Geometry: final body of the model. Coordinates: model frame, mm. A direction names the side the tool comes from. Coordinates: 2 decimals unless noted, no trailing zeros. Loops run counter-clockwise (first coordinate to the right, second up) from the corner with the lowest first, then second, coordinate; pieces in that order, holes last. Notation, with made-up numbers: (9.5, -1) - (16.5, -1) arc R21 cw to (16.5, 20) - close; hole circle Ø10 at (-11.5, 36). An arc over 180 degrees is marked (long way). Put each result on its own line as item: value. Start each with the question number.
1) Draft query along Y for faces 1 (the cylindrical face through (-23, -2, -5)), 2 (the flat face through (4, -130, -2)), 3 (the cylindrical face through (-25.479, -79.547, -16.284)). Return one class per face: +Y half, -Y half, draft (parallel to the pull), parting line (faces both ways), or undercut.
2) Section D-D on x = -15.5. Output: boundary loops of the cut face in (y, z), and give its area (3 significant figures).
3) Section C-C on y = -98. Output: boundary loops of the cut face in (x, z), and give its area (3 significant figures).
4) Section B-B on z = -17. Count the separate pieces of the cut face and the enclosed holes in it, and give its area (3 significant figures).
5) Contact query for flat-ended pins moving along their axis: pin 1 Ø19 at (x, y) = (-4.5, 22.5) entering from -Z; pin 2 Ø0.9 at (x, y) = (26, -9) entering from +Z; pin 3 Ø6 at (x, z) = (-18.5, -14) entering from +Y; pin 4 Ø0.9 at (x, y) = (-25.5, 12) entering from +Z. Output: stop coordinate, or through.
6) Section A-A on y = -19.5. Output: boundary loops of the cut face in (x, z).
7) Reachability of faces 4 (the flat face through (27, 2, -24)), 5 (the cylindrical face through (25.5, 115.5, -16.9)), 6 (the cylindrical face through (23, 2, -5)) from +Z, -Z, +X, -X, +Y, -Y: full face, straight path, thin tool, end or side. Return the list, or none.
8) Material intervals for line 1 along Y through (x, z) = (-25.05, -17); line 2 along X through (y, z) = (-66.5, -29.5); line 3 along Z through (x, y) = (-10, 23), sorted ascending. Write a range as from..to.
```python
from build123d import *

# Parameters (mm, degrees)
SKETCH1_W                      = 54
SKETCH1_H                      = 260
BASE_FLANGE1_DEPTH             = 3
EDGE_FLANGE1_STRIP_W           = 22
EDGE_FLANGE1_STRIP_H           = 3
EDGE_FLANGE1_STRIP_CUT_DEPTH   = 260
EDGE_FLANGE1_STRIP_2_W         = 22
EDGE_FLANGE1_STRIP_2_H         = 3
EDGE_FLANGE1_STRIP_CUT_2_DEPTH = 260
EDGE_FLANGE1_DEPTH             = 260
EDGE_FLANGE1_BEND_DEPTH        = 260
CUT_EXTRUDE1_DEPTH             = 145.817126059
SKETCH20_R                     = 5.5
CUT_EXTRUDE2_DEPTH             = 145.817126059


# Sheet-metal steps are written as plain solids
with BuildPart() as part:
    # Sketch1 → Base-Flange1 (new body)
    with BuildSketch(Plane.XY):
        Rectangle(SKETCH1_W, SKETCH1_H)
    extrude(amount=-BASE_FLANGE1_DEPTH)

    # Edge-Flange1 strip (across the edge) → Edge-Flange1 strip cut (cut)
    with BuildSketch(Plane(origin=(27, 130, -3), x_dir=(-1, 0, 0), z_dir=(0, -1, 0))):
        with Locations((-3, -1.5)):
            Rectangle(EDGE_FLANGE1_STRIP_W, EDGE_FLANGE1_STRIP_H)
    extrude(amount=EDGE_FLANGE1_STRIP_CUT_DEPTH, mode=Mode.SUBTRACT)

    # Edge-Flange1 strip 2 (across the edge) → Edge-Flange1 strip cut 2 (cut)
    with BuildSketch(Plane(origin=(-27, -130, -3), x_dir=(1, 0, 0), z_dir=(0, 1, 0))):
        with Locations((-3, -1.5)):
            Rectangle(EDGE_FLANGE1_STRIP_2_W, EDGE_FLANGE1_STRIP_2_H)
    extrude(amount=EDGE_FLANGE1_STRIP_CUT_2_DEPTH, mode=Mode.SUBTRACT)

    # Edge-Flange1 section (across the edge) → Edge-Flange1 (add)
    with BuildSketch(Plane(origin=(27, 130, -3), x_dir=(-1, 0, 0), z_dir=(0, -1, 0))):
        with BuildLine():
            Line((0, 5), (0, 31))
            Line((0, 31), (3, 31))
            Line((3, 31), (3, 5))
            ThreePointArc((3, 5), (4.464466094, 1.464466094), (8, 0))
            Line((8, 0), (8, -3))
            ThreePointArc((8, -3), (2.343145751, -0.656854249), (0, 5))
        make_face()
    extrude(amount=EDGE_FLANGE1_DEPTH)

    # Edge-Flange1 section 2 (across the edge) → Edge-Flange1 bend (add)
    with BuildSketch(Plane(origin=(-27, -130, -3), x_dir=(1, 0, 0), z_dir=(0, 1, 0))):
        with BuildLine():
            Line((0, 5), (0, 31))
            Line((0, 31), (3, 31))
            Line((3, 31), (3, 5))
            ThreePointArc((3, 5), (4.464466094, 1.464466094), (8, 0))
            Line((8, 0), (8, -3))
            ThreePointArc((8, -3), (2.343145751, -0.656854249), (0, 5))
        make_face()
    extrude(amount=EDGE_FLANGE1_BEND_DEPTH)

    # Sketch18 → Cut-Extrude1 (cut, through all)
    with BuildSketch(Plane(origin=(27, 0, 0), x_dir=(0, 0, -1), z_dir=(1, 0, 0))):
        with BuildLine():
            Line((11.5, -60), (11.5, 110))
            ThreePointArc((11.5, 110), (17, 115.5), (22.5, 110))
            Line((22.5, 110), (22.5, -60))
            ThreePointArc((22.5, -60), (17, -65.5), (11.5, -60))
        make_face()
    extrude(amount=-CUT_EXTRUDE1_DEPTH, mode=Mode.SUBTRACT)

    # Sketch20 → Cut-Extrude2 (cut, through all)
    with BuildSketch(Plane(origin=(27, 0, 0), x_dir=(0, 0, -1), z_dir=(1, 0, 0))):
        with Locations((17, -115)):
            Circle(SKETCH20_R)
        with Locations((17, -85)):
            Circle(SKETCH20_R)
    extrude(amount=-CUT_EXTRUDE2_DEPTH, mode=Mode.SUBTRACT)


solid = part.part
```
Answer block:
1. face 1: draft
1. face 2: -Y half
1. face 3: undercut
2. outline: (-130, -3) - (130, -3) - (130, 0) - (-130, 0) - close
2. area: 780 mm²
3. outline: (-27, -34) - (-24, -34) - (-24, -8) arc R5 cw to (-19, -3) - (19, -3) arc R5 cw to (24, -8) - (24, -34) - (27, -34) - (27, -8) arc R8 ccw to (19, 0) - (-19, 0) arc R8 ccw to (-27, -8) - close
3. area: 331 mm²
4. separate pieces: 8
4. enclosed holes: 0
4. area: 342 mm²
5. pin 1: stops at z = -3
5. pin 2: stops at z = -3.41
5. pin 3: passes through
5. pin 4: stops at z = -2.77
6. outline: (-27, -34) - (-24, -34) - (-24, -22.5) - (-27, -22.5) - close; (-27, -11.5) - (-24, -11.5) - (-24, -8) arc R5 cw to (-19, -3) - (19, -3) arc R5 cw to (24, -8) - (24, -11.5) - (27, -11.5) - (27, -8) arc R8 ccw to (19, 0) - (-19, 0) arc R8 ccw to (-27, -8) - close; (24, -34) - (27, -34) - (27, -22.5) - (24, -22.5) - close
7. face 4: +Z, -Z, +X, +Y, -Y
7. face 5: +X, -X
7. face 6: -Z, +Y, -Y
8. line 1: y = -130..-120.5, -109.5..-90.5, -79.5..-65.5, 115.5..130
8. line 2: x = -27..-24, 24..27
8. line 3: z = -3..0
